```python
from build123d import *

# Parameters (mm, degrees)
SKETCH1_W           = 425.45
SKETCH1_H           = 349.25
BOSS_EXTRUDE1_DEPTH = 133.35
SKETCH3_W           = 101.611122636
SKETCH3_H           = 27.910351282
CUT_EXTRUDE1_DEPTH  = 7.62
SKETCH4_R           = 6.35
BOSS_EXTRUDE2_DEPTH = 7.62
SKETCH5_R           = 7.62
BOSS_EXTRUDE3_DEPTH = 5.08
FILLET1_SIZE        = 1.27
SKETCH7_R           = 6.35
BOSS_EXTRUDE4_DEPTH = 2.54
SKETCH8_R           = 6.35
BOSS_EXTRUDE5_DEPTH = 7.62


with BuildPart() as part:
    # Sketch1 → Boss-Extrude1 (new body)
    with BuildSketch(Plane(origin=(0, 0, 0), x_dir=(1, 0, 0), z_dir=(0, 1, 0))):
        Rectangle(SKETCH1_W, SKETCH1_H)
    extrude(amount=BOSS_EXTRUDE1_DEPTH)

    # Sketch3 → Cut-Extrude1 (cut)
    with BuildSketch(Plane.XY.offset(174.625)):
        with Locations((50.805561318, 100.690740625)):
            Rectangle(SKETCH3_W, SKETCH3_H)
    extrude(amount=-CUT_EXTRUDE1_DEPTH, mode=Mode.SUBTRACT)

    # Sketch4 → Boss-Extrude2 (add)
    with BuildSketch(Plane.XY.offset(174.625)):
        with Locations(Location((3.924893149, 40.875369667, 0), (0, 0, 180))):
            Circle(SKETCH4_R)
    extrude(amount=BOSS_EXTRUDE2_DEPTH)

    # Sketch5 → Boss-Extrude3 (add)
    with BuildSketch(Plane.XY.offset(174.625)):
        with Locations(Location((41.429427684, 29.10069022, 0), (0, 0, 180))):
            Circle(SKETCH5_R)
    extrude(amount=BOSS_EXTRUDE3_DEPTH)

    # Fillet1
    # a fillet whose section is not a circle: 1.27 mm, written as the material it takes off along each edge
    with BuildSketch(Plane(origin=(41.429427684, 29.10069022, 179.705), x_dir=(-1, 0, 0), z_dir=(0, 1, 0))) as fillet1_piece_1:
        with BuildLine():
            Bezier((7.62, -FILLET1_SIZE), (7.62, 0), (7.62 - FILLET1_SIZE, 0), weights=[1, 3.535533906, 1])
            Line((7.62 - FILLET1_SIZE, 0), (7.62, 0))
            Line((7.62, 0), (7.62, -FILLET1_SIZE))
        make_face()
    revolve(axis=Axis((41.429427684, 29.10069022, 179.705), (0, 0, 1)), mode=Mode.SUBTRACT)

    # Sketch7 → Boss-Extrude4 (add)
    with BuildSketch(Plane.XY.offset(179.705)):
        with Locations(Location((41.536592477, 29.04493903, 0), (0, 0, 241.893573302))):
            Circle(SKETCH7_R)
    extrude(amount=BOSS_EXTRUDE4_DEPTH)

    # Sketch8 → Boss-Extrude5 (add)
    with BuildSketch(Plane.XY.offset(174.625)):
        with Locations(Location((108.588710457, 40.1644131, 0), (0, 0, 180))):
            Circle(SKETCH8_R)
    extrude(amount=BOSS_EXTRUDE5_DEPTH)


solid = part.part
```
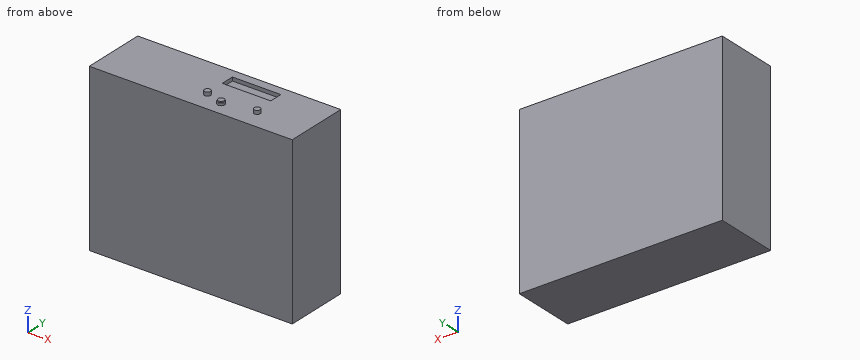
Work out the finished part from the listing and answer in its coordinate system (mm). Coordinates: 2 decimals unless noted, no trailing zeros. Write each loop counter-clockwise with the first axis right and the second up, starting at its lowest first coordinate (ties: lowest second). Pieces come first, ordered by that corner, then holes. Notation, with made-up numbers: (41, 84) - (62, 84) arc R7 ccw to (62, 95) - close; hole circle Ø9 at (46.5, 66). An arc over 180 degrees is marked (long way). Answer as a JSON object with one key per item and string values.
Q1. Find section C-C (y = 8.5). Write down the section's boundary in (x, z) (3 decimals), plus the area to 3 significant figures.
Results list:
{"outline": "(-212.725, -174.625) - (212.725, -174.625) - (212.725, 174.625) - (-212.725, 174.625) - close", "area": "149,000 mm^2"}
Q2. Consider L1, parallel to Z at x = -84, y = 69 (3 decimals). Determine where the line is inside the solid, lowest interval first. Write a range as from..to.
Results list:
{"L1": "z = -174.625..174.625"}
Q3. Find section B-B (x = 155). Write down the section's boundary in (y, z) (3 decimals).
Results list:
{"outline": "(0, -174.625) - (133.35, -174.625) - (133.35, 174.625) - (0, 174.625) - close"}
Q4. Find section A-A (y = 110). Write down the section's boundary in (x, z) (3 decimals), plus the area to 3 significant figures.
Results list:
{"outline": "(-212.725, -174.625) - (212.725, -174.625) - (212.725, 174.625) - (101.611, 174.625) - (101.611, 167.005) - (0, 167.005) - (0, 174.625) - (-212.725, 174.625) - close", "area": "148,000 mm^2"}
Q5. Given pin 1 Ø8.5 at (x, y) = (27.5, 98) entering from +Z (3 decimals); pin 2 Ø10 at (x, y) = (-49.5, 94.5) entering from +Z (3 decimals), each flat-ended and moving along its own axis, determine where each tip first touches the part or whether it passes through.
Results list:
{"pin 1": "stops at z = 167.005", "pin 2": "stops at z = 174.625"}
